Autodesk Inventor part; units mm, degrees
ref_plane "YZ Plane" through (0, 0, 0) normal (1, 0, 0) x (0, 1, 0)
ref_plane "XZ Plane" through (0, 0, 0) normal (0, 1, 0) x (-1, 0, 0)
ref_plane "XY Plane" through (0, 0, 0) normal (0, 0, 1) x (1, 0, 0)
sketch "Sketch1" plane through (0, 0, 0) normal (0, 0, 1) x (1, 0, 0)
  line L0 (0, 0) -> (135, 0)
  line L1 (135, 0) -> (135, 42)
  line L2 (135, 42) -> (0, 42)
  line L3 (0, 42) -> (0, 0)
  dimension "d0" = 135
  dimension "d1" = 42
extrude "Extrusion1" add sketch "Sketch1" along normal blind 23.3
fillet "Fillet1" radius 2 12 edges at (67.5, 42, 23.3) (0, 42, 11.65) (67.5, 42, 0) (0, 21, 23.3) (67.5, 0, 23.3) (0, 0, 11.65) (0, 21, 0) (135, 21, 23.3) (135, 0, 11.65) (135, 21, 0) (135, 42, 11.65) (67.5, 0, 0)
sketch "Sketch2" plane through (0, 0, 23.3) normal (0, 0, 1) x (1, 0, 0)
  line L0 (112.9507, 4.761) -> (47.847, 4.761) construction
  line L1 (47.847, 4.761) -> (47.847, 21.3737) construction
  line L2 (47.847, 21.3737) -> (112.9507, 21.3737) construction
  line L3 (112.9507, 21.3737) -> (112.9507, 4.761) construction
sketch "Sketch3" plane through (135, 2, 2) normal (1, 0, 0) x (0, 0, -1)
  line L0 (-19.3, -2) -> (0, -2)
  line L1 (0, 40) -> (-19.3, 40)
  circle A0 centre (-8.3, 0) radius 2
  circle A1 centre (-4.3, 0) radius 2
  circle A2 centre (-9.3, 39) radius 1
  circle A3 centre (-7.3, 39) radius 1
  circle A4 centre (-5.3, 39) radius 1
  circle A5 centre (-3.3, 39) radius 1
  line L2 (-21.3, 38) -> (-21.3, 0)
  point P0 (2, -2)
  dimension "d5" = 4
  dimension "d6" = 4
  dimension "d7" = 2
  dimension "d8" = 2
  dimension "d9" = 2
  dimension "d10" = 2
  dimension "d11" = 12
  dimension "d12" = 13
extrude "Extrusion2" add sketch "Sketch3" along normal blind 15 and the other way blind 3 contours A0 | A1 | A5 | A4 | A3 | A2
properties part number "DriveBattery" material "ABS Plastic"
Work out the finished part from the listing and answer in its coordinate system (mm). Coordinates: 2 decimals unless noted, no trailing zeros. Loops run counter-clockwise (first coordinate to the right, second up) from the corner with the lowest first, then second, coordinate; pieces in that order, holes last.
1) Consider probe 1 along X at (y, z) = (13.5, 1.75); probe 2 along Y at (x, z) = (136, 11.5); probe 3 along X at (y, z) = (27, 22). Determine where each line is inside the solid, lowest interval first.
Results:
probe 1: x = 0.02 to 134.98
probe 2: y = 0.4 to 3.6, 40.02 to 41.98
probe 3: x = 0.13 to 134.87
2) Section B-B (y = 18) is taken. Give the vertices of the cut face in (x, z), plus the area to 3 significant figures.
Results:
outline: (0, 2) arc R2 ccw to (2, 0) - (133, 0) arc R2 ccw to (135, 2) - (135, 21.3) arc R2 ccw to (133, 23.3) - (2, 23.3) arc R2 ccw to (0, 21.3) - close
area: 3,140 mm2
3) Section C-C (z = 14) is taken. Give the vertices of the cut face in (x, y), plus the area to 3 significant figures.
Results:
outline: (0, 2) arc R2 ccw to (2, 0) - (133, 0) arc R2 ccw to (135, 2) - (135, 40) arc R2 ccw to (133, 42) - (2, 42) arc R2 ccw to (0, 40) - close
area: 5,670 mm2
4) Flat-ended cylindrical pins translate along their axes: pin 1 (8 mm diameter, centred on x = 36.5, y = 26, fed in from -Z); pin 2 (9.5 mm diameter, centred on y = 19.5, z = 8, fed in from +X). Find the tip coordinate at first contact, or state that the pin passes through.
Results:
pin 1: stops at z = 0
pin 2: stops at x = 135
5) For a pull along Y with two mould halves and no side action, classify faces 1 (the flat face through (68, 42, 12)), 2 (the flat face through (150, 2, 10)), 3 (the flat face through (135, 21, 12)) as +Y half, -Y half, draft (parallel to the pull), parting line (faces both ways), or undercut.
Results:
face 1: +Y half
face 2: draft
face 3: undercut
